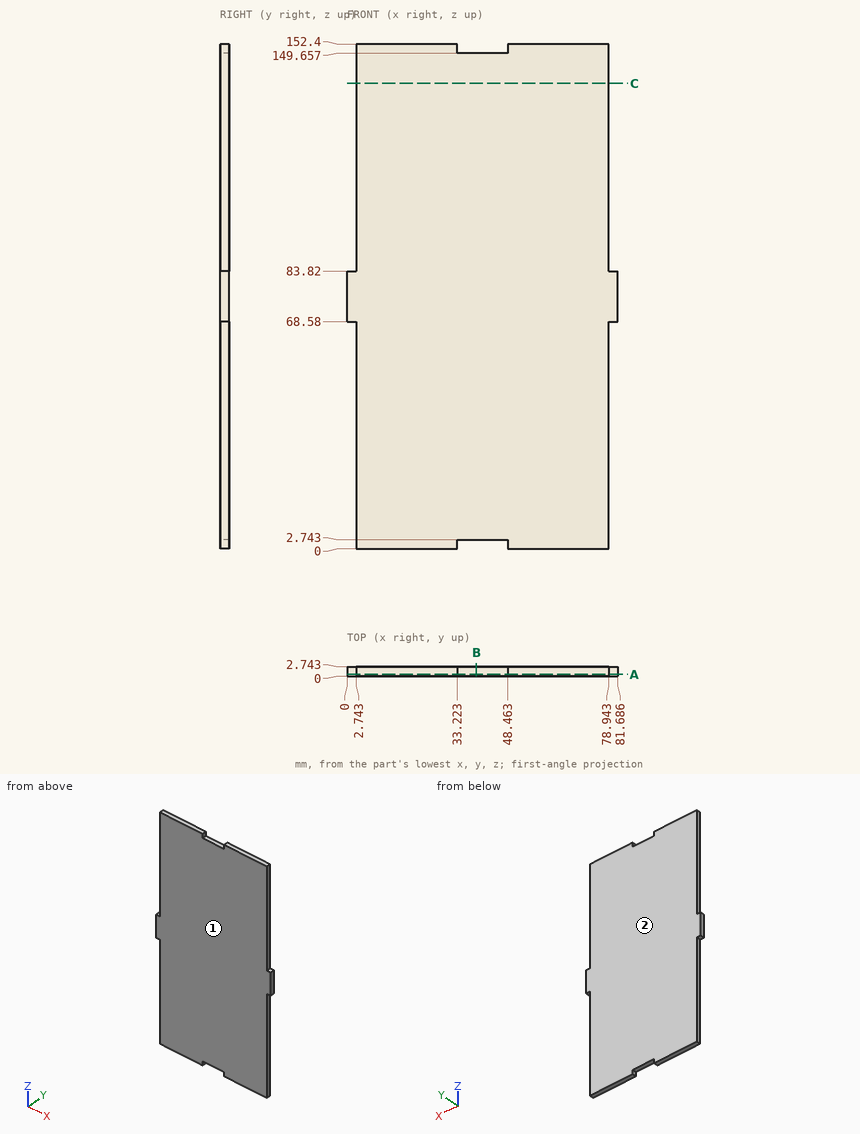
Job drawing, mm, ordinate dimensions from the low corner. One solid piece. Round coordinates to 2 decimals unless told otherwise and drop trailing zeros. Write each loop counter-clockwise with the first axis right and the second up, starting at its lowest first coordinate (ties: lowest second). Pieces come first, ordered by that corner, then holes.
1) Drill centre lines: probe 1 along Z at (x, y) = (47, 1.5); probe 2 along X at (y, z) = (1, 115). Where is each one in solid material? Low to high.
2) Mould opens along Y. For the marked faces 1 and 2 say: +Y half, -Y half, draft (parallel to the pull), parting line (faces both ways), or undercut.
3) Band-saw the part on C-C, the plane z = 140.5. List the corners of the cut face in (x, y), and give its area (3 significant figures).
4) Pin check, flat tips, straight feed: pin 1 (0.8 mm diameter, centred on y = 1.5, z = 34.5, fed in from +X); pin 2 (1.4 mm diameter, centred on x = 41.5, y = 1.5, fed in from +Z); pin 3 (1.4 mm diameter, centred on y = 1.5, z = 151.5, fed in from -X). Stop position of each tip, or through.
5) Band-saw the part on B-B, the plane x = 39. List the corners of the cut face in (y, z), and give its area (3 significant figures).
6) Band-saw the part on A-A, the plane y = 0.5. List the corners of the cut face in (x, z), and give its area (3 significant figures).
Ans:
1. probe 1: z = 2.74 to 149.66
1. probe 2: x = 2.74 to 78.94
2. face 1: -Y half
2. face 2: +Y half
3. outline: (2.74, 0) - (78.94, 0) - (78.94, 2.74) - (2.74, 2.74) - close
3. area: 209 mm2
4. pin 1: stops at x = 78.94
4. pin 2: stops at z = 149.66
4. pin 3: stops at x = 2.74
5. outline: (0, 2.74) - (2.74, 2.74) - (2.74, 149.66) - (0, 149.66) - close
5. area: 403 mm2
6. outline: (0, 68.58) - (2.74, 68.58) - (2.74, 0) - (33.22, 0) - (33.22, 2.74) - (48.46, 2.74) - (48.46, 0) - (78.94, 0) - (78.94, 68.58) - (81.69, 68.58) - (81.69, 83.82) - (78.94, 83.82) - (78.94, 152.4) - (48.46, 152.4) - (48.46, 149.66) - (33.22, 149.66) - (33.22, 152.4) - (2.74, 152.4) - (2.74, 83.82) - (0, 83.82) - close
6. area: 11,600 mm2
